from build123d import *

# Parameters (mm, degrees)
VYSUNOUT1_DEPTH = 6
SKICA3_R        = 6
VYSUNOUT2_DEPTH = 1
SKICA4_R        = 4
VYSUNOUT3_DEPTH = 8
ZKOSIT1_SIZE    = 0.8
ZAOBLIT1_R      = 0.2
ZAOBLIT2_R      = 0.2


with BuildPart() as part:
    # Skica1 → Vysunout1 (new body)
    with BuildSketch(Plane.XY):
        Polygon((6, 3.464101615), (0, 6.92820323), (-6, 3.464101615), (-6, -3.464101615), (0, -6.92820323), (6, -3.464101615), align=None)
    extrude(amount=VYSUNOUT1_DEPTH)

    # Skica2 → Odebrat otočením1 (revolve, cut)
    with BuildSketch(Plane(origin=(0, 0, 0), x_dir=(1, 0, 0), z_dir=(0, 1, 0))):
        Polygon((6, 0), (28.392304845, 0), (28.392304845, -6), align=None)
    revolve(axis=Axis((0, 0, 0), (0, 0, 1)), mode=Mode.SUBTRACT)

    # Skica3 → Vysunout2 (add)
    with BuildSketch(Plane.XY.offset(6)):
        Circle(SKICA3_R)
    extrude(amount=VYSUNOUT2_DEPTH)

    # Skica4 → Vysunout3 (add)
    with BuildSketch(Plane.XY.offset(7)):
        Circle(SKICA4_R)
    extrude(amount=VYSUNOUT3_DEPTH)

    # Zkosit1
    zkosit1_edges = [part.edges().sort_by_distance(p)[0] for p in [
        (-4, 0, 15),
    ]]
    chamfer(zkosit1_edges, length=ZKOSIT1_SIZE)

    # Skica6 → Odebrat otočením2 (revolve, cut)
    with BuildSketch(Plane(origin=(0, 0, 0), x_dir=(1, 0, 0), z_dir=(0, 1, 0))):
        Polygon((0, -11.464101615), (2, -12), (2, -15), (0, -15), align=None)
    revolve(axis=Axis((0, 0, 15), (0, 0, -1)), mode=Mode.SUBTRACT)

    # Zaoblit1
    zaoblit1_edges = [part.edges().sort_by_distance(p)[0] for p in [
        (-2, 0, 12),
    ]]
    fillet(zaoblit1_edges, radius=ZAOBLIT1_R)

    # Skica7 → Odebrat otočením3 (revolve, cut)
    with BuildSketch(Plane(origin=(0, 0, 0), x_dir=(1, 0, 0), z_dir=(0, 1, 0)), mode=Mode.PRIVATE) as odebrat_oto_en_m3_sk:
        Polygon((4, -7), (3.25, -7.433012702), (4, -7.866025404), align=None)
    revolve(odebrat_oto_en_m3_sk.sketch.rotate(Axis((0, 0, 0), (0, 0, 1)), 180), axis=Axis((0, 0, 0), (0, 0, 1)), mode=Mode.SUBTRACT)

    # Zaoblit2
    zaoblit2_edges = [part.edges().sort_by_distance(p)[0] for p in [
        (3.25, 0, 7.433012702),
        (4, 0, 7),
    ]]
    fillet(zaoblit2_edges, radius=ZAOBLIT2_R)


solid = part.part
Build history of the part. All positions in model axes, mm. A direction names the side the tool comes from. Round coordinates to 2 decimals unless told otherwise and drop trailing zeros. Write each loop counter-clockwise with the first axis right and the second up, starting at its lowest first coordinate (ties: lowest second). Pieces come first, ordered by that corner, then holes. Notation, with made-up numbers: M -15.5,21 L 2.5,21 A24 cw 2.5,33 Z; hole C 75.5,30 d11. An arc over 180 degrees is marked long. Use CSV: the item, a comma, the result in double quotes.
1. Flat gauge pins, fed straight in: pin 1 (0.9 mm diameter, centred on x = -4.5, y = 4, fed in from +Z); pin 2 (5 mm diameter, centred on y = 4, z = 13.5, fed in from +X); pin 3 (2.5 mm diameter, centred on x = 0, y = 0, fed in from +Z); pin 4 (1.5 mm diameter, centred on y = 5, z = 13, fed in from -X). Where does each tip first touch, or does it go through?
Reply:
pin 1,"stops at z = 7"
pin 2,"stops at x = 3.71"
pin 3,"stops at z = 11.8"
pin 4,"passes through"
2. Tool access for faces 4 (the face through (5.4, 3.1, 0.06)), 5 (the face through (0, -6.2, 6)), 6 (the face through (5.4, -3.2, 6)), 7 (the face through (-5.38, 3.12, 0.06)), 8 (the face through (-5.994, 0.264, 6.493)): list every direction of +Z, -Z, +X, -X, +Y, -Y with a clear straight run to the whole face (end or side of a thin tool).
Reply:
face 4,"-Z, +X, +Y"
face 5,"+Z, -Y"
face 6,"+Z, +X, -Y"
face 7,"-Z, -X, +Y"
face 8,"+Z"
3. Saw through at A-A (z = 1.25). Give the cut face in (x, y).
Reply:
outline,"M -6,-3.46 L 0,-6.93 L 6,-3.46 L 6,3.46 L 0,6.93 L -6,3.46 Z"
4. Two-plate mould, pull along Z, no slides. Class faces 1 (the face through (-0.02, -6.22, 0.06)), 2 (the face through (-3.042, -5.172, 2.958)), 3 (the face through (-5.4, 3, 6)): +Z half, -Z half, draft (parallel to the pull), parting line (faces both ways), or undercut.
Reply:
face 1,"-Z half"
face 2,"draft"
face 3,"+Z half"
5. Wall check: probe 1 along Y at (x, z) = (0, 13.15); probe 2 along Y at (x, z) = (0, 14.25); probe 3 along Z at (x, y) = (0.25, 5). Give the ranges that are in metal, low to high. Write a range as from..to.
Reply:
probe 1,"y = -4..-2, 2..4"
probe 2,"y = -3.95..-2, 2..3.95"
probe 3,"z = 0..7"
